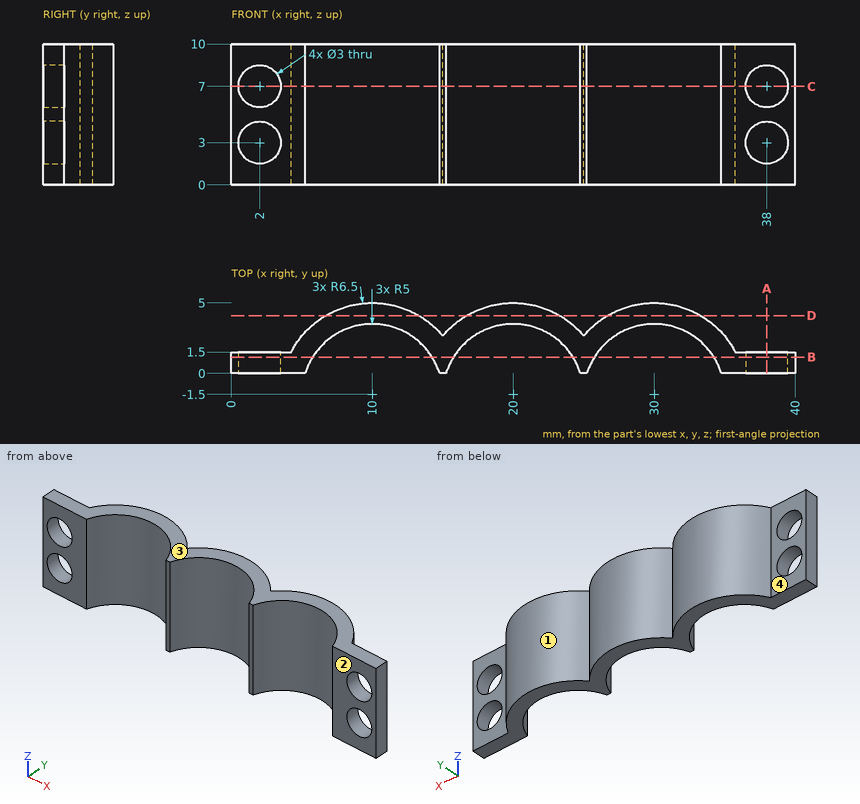
Job drawing, mm, ordinate dimensions from the low corner. One solid piece. A direction names the side the tool comes from. Round coordinates to 2 decimals unless told otherwise and drop trailing zeros. Write each loop counter-clockwise with the first axis right and the second up, starting at its lowest first coordinate (ties: lowest second). Pieces come first, ordered by that corner, then holes. Notation, with made-up numbers: M -7,77 L 19,77 A14 cw 19,84 Z; hole C -17,70 d5. An arc over 180 degrees is marked long. Return JSON: item names as keys, results as strings. Group by question number.
(1) Two-plate mould, pull along X, no slides. Class the marked faces 1 and 2: +X half, -X half, draft (parallel to the pull), parting line (faces both ways), or undercut.
(2) Saw through at A-A on x = 38. Write the cut outline in (y, z).
(3) Which spindle directions (+Z, -Z, +X, -X, +Y, -Y) get a long thin tool onto all of the face, cutting with end or side? Do the marked faces 3 and 4. Say none if no direction does.
(4) Saw through at C-C on z = 7. Write the cut outline in (x, y), then the cut area to 3 significant figures.
(5) Drill centre lines: probe 1 along X at (y, z) = (3.95, 3); probe 2 along X at (y, z) = (3.6, 3); probe 3 along X at (y, z) = (0.6, 5.25). Where is each one in solid material? Low to high.
(6) Saw through at B-B on y = 1.15. Write the cut outline in (x, z).
(7) Pin check, flat tips, straight feed: pin 1 Ø1 at (x, z) = (10, 8) entering from -Y; pin 2 Ø3.5 at (x, z) = (38, 7) entering from +Y; pin 3 Ø1 at (x, z) = (22.5, 6.5) entering from +Y. Stop position of each tip, or through.
(8) Saw through at D-D on y = 4.1. Write the cut outline in (x, z).
Returned:
{
 "1": {"face 1": "undercut", "face 2": "draft"},
 "2": {"outline": "M 0,0 L 1.5,0 L 1.5,1.5 L 0,1.5 Z; M 0,4.5 L 1.5,4.5 L 1.5,5.5 L 0,5.5 Z; M 0,8.5 L 1.5,8.5 L 1.5,10 L 0,10 Z"},
 "3": {"face 3": "+Z, +X, -X, +Y, -Y", "face 4": "+Z, -Z, -X, +Y"},
 "4": {"outline": "M 0,0 L 0.5,0 L 0.5,1.5 L 0,1.5 Z; M 3.5,0 L 5.23,0 A5 cw 14.77,0 L 15.23,0 A5 cw 24.77,0 L 25.23,0 A5 cw 34.77,0 L 36.5,0 L 36.5,1.5 L 35.77,1.5 A6.5 ccw 25,2.65 A6.5 ccw 15,2.65 A6.5 ccw 4.23,1.5 L 3.5,1.5 Z; M 39.5,0 L 40,0 L 40,1.5 L 39.5,1.5 Z", "area": "62.0 mm²"},
 "5": {"probe 1": "6.46 to 13.54, 16.46 to 23.54, 26.46 to 33.54", "probe 2": "5.97 to 14.03, 15.97 to 24.03, 25.97 to 34.03", "probe 3": "0 to 5.46, 14.54 to 15.46, 24.54 to 25.46, 34.54 to 40"},
 "6": {"outline": "M 0,0 L 5.76,0 L 5.76,10 L 0,10 Z; M 14.24,0 L 15.76,0 L 15.76,10 L 14.24,10 Z; M 24.24,0 L 25.76,0 L 25.76,10 L 24.24,10 Z; M 34.24,0 L 40,0 L 40,10 L 34.24,10 Z; hole C 2,3 d3; hole C 2,7 d3; hole C 38,3 d3; hole C 38,7 d3"},
 "7": {"pin 1": "y = 3.47", "pin 2": "y = 1.5", "pin 3": "y = 4.68"},
 "8": {"outline": "M 6.7,0 L 13.3,0 L 13.3,10 L 6.7,10 Z; M 16.7,0 L 23.3,0 L 23.3,10 L 16.7,10 Z; M 26.7,0 L 33.3,0 L 33.3,10 L 26.7,10 Z"}
}
